```python
from build123d import *

# Parameters (mm, degrees)
W_TOP_DEPTH                  = 3.175
SKETCH3_W                    = 16.4
SKETCH3_H                    = 12
SKETCH3_W_2                  = 35.6
SKETCH3_H_2                  = 4.6
A_HOLDERS_DEPTH              = 5.5
A_CLAMP_DEPTH                = 2
SKETCH12_R                   = 1.35
SKETCH12_W                   = 25
SKETCH12_H                   = 45.3
A_HOLES_DEPTH                = 3.175
A_HOLES_START                = 1
A_HOLES_GUIDE_DEPTH          = 1.5
SKETCH15_R                   = 3.175
TENDON_HOLES_DEPTH           = 3.175
SKETCH16_R                   = 4.675
SKETCH16_R_2                 = 3.175
TUBE_SUPPORT_DEPTH           = 5
SKETCH19_R                   = 3.175
THICKNESS_COMPENSATION_DEPTH = 2.2
SKETCH18_R                   = 5
GEAR_PLACEMENTS_DEPTH        = 1.25
SKETCH20_R                   = 2.155
SCREW_HOLES_DEPTH            = 5.375
SKETCH21_R                   = 3.275
STANDOFF_HOLE_DEPTH          = 2.7


with BuildPart() as part:
    # Sketch1 → w_top (new body)
    with BuildSketch(Plane(origin=(0, 0, 0), x_dir=(1, 0, 0), z_dir=(0, 1, 0))):
        with BuildLine():
            Line((-48, -35), (-48, 30))
            ThreePointArc((-48, 30), (-42.142135624, 44.142135624), (-28, 50))
            Line((-28, 50), (28, 50))
            ThreePointArc((28, 50), (42.142135624, 44.142135624), (48, 30))
            Line((48, 30), (48, -35))
            ThreePointArc((48, -35), (42.142135624, -49.142135624), (28, -55))
            Line((28, -55), (-28, -55))
            ThreePointArc((-28, -55), (-42.142135624, -49.142135624), (-48, -35))
        make_face()
    extrude(amount=W_TOP_DEPTH)

    # Sketch3 → a_holders (add)
    with BuildSketch(Plane(origin=(0, 3.175, 0), x_dir=(1, 0, 0), z_dir=(0, 1, 0))):
        Polygon((0.5, -24.5), (0.5, -34), (41.1, -34), (41.1, -24.5), (33, -24.5), (33, -8.5), (8.6, -8.5), (8.6, -24.5), align=None)
        with Locations((20.8, -18.5)):
            Rectangle(SKETCH3_W, SKETCH3_H, mode=Mode.SUBTRACT)
        with Locations((20.8, -29.25)):
            Rectangle(SKETCH3_W_2, SKETCH3_H_2, mode=Mode.SUBTRACT)
        Polygon((8.6, 26.5), (-8.6, 26.5), (-8.6, 10.5), (-33, 10.5), (-33, 26.5), (-41.1, 26.5), (-41.1, 36), (41.1, 36), (41.1, 26.5), (33, 26.5), (33, 10.5), (8.6, 10.5), align=None)
        with Locations((20.8, 20.5)):
            Rectangle(SKETCH3_W, SKETCH3_H, mode=Mode.SUBTRACT)
        with Locations((-20.8, 20.5)):
            Rectangle(SKETCH3_W, SKETCH3_H, mode=Mode.SUBTRACT)
        with Locations((-20.8, 31.25)):
            Rectangle(SKETCH3_W_2, SKETCH3_H_2, mode=Mode.SUBTRACT)
        with Locations((20.8, 31.25)):
            Rectangle(SKETCH3_W_2, SKETCH3_H_2, mode=Mode.SUBTRACT)
    extrude(amount=A_HOLDERS_DEPTH)

    # Sketch14 → a_clamp (add)
    with BuildSketch(Plane(origin=(0, 8.675, 0), x_dir=(1, 0, 0), z_dir=(0, 1, 0))):
        Polygon((-35.6, 33.55), (-35.6, 36), (-41.1, 36), (-41.1, 26.5), (-35.6, 26.5), (-35.6, 28.95), (-38.6, 28.95), (-38.6, 33.55), align=None)
        Polygon((6, -24.5), (0.5, -24.5), (0.5, -34), (6, -34), (6, -31.55), (3, -31.55), (3, -26.95), (6, -26.95), align=None)
        Polygon((-3, 33.55), (-6, 33.55), (-6, 36), (6, 36), (6, 33.55), (3, 33.55), (3, 28.95), (6, 28.95), (6, 26.5), (-6, 26.5), (-6, 28.95), (-3, 28.95), align=None)
        Polygon((38.6, 33.55), (35.6, 33.55), (35.6, 36), (41.1, 36), (41.1, 26.5), (35.6, 26.5), (35.6, 28.95), (38.6, 28.95), align=None)
        Polygon((35.6, -26.95), (35.6, -24.5), (41.1, -24.5), (41.1, -34), (35.6, -34), (35.6, -31.55), (38.6, -31.55), (38.6, -26.95), align=None)
    extrude(amount=A_CLAMP_DEPTH)

    # Sketch12 → a_holes (cut)
    with BuildSketch(Plane(origin=(0, 3.175, 0), x_dir=(1, 0, 0), z_dir=(0, 1, 0))):
        with Locations((-28.8, -47.8)):
            Circle(SKETCH12_R)
        with Locations((-11.8, -47.8)):
            Circle(SKETCH12_R)
        with Locations((-35.3, -24.5)):
            Circle(SKETCH12_R)
        with Locations((-5.3, -24.5)):
            Circle(SKETCH12_R)
        with Locations((-20.3, -22.45)):
            Rectangle(SKETCH12_W, SKETCH12_H)
    extrude(amount=-A_HOLES_DEPTH, mode=Mode.SUBTRACT)

    # Sketch13 → a_holes guide (cut)
    with BuildSketch(Plane.XZ.offset(A_HOLES_START)):
        with BuildLine():
            Line((-31.6, 47.8), (-31.6, 45.1))
            Line((-31.6, 45.1), (-26, 45.1))
            Line((-26, 45.1), (-26, 47.8))
            ThreePointArc((-26, 47.8), (-28.8, 50.6), (-31.6, 47.8))
        make_face()
        with BuildLine():
            Line((-35.3, 27.3), (-32.8, 27.3))
            Line((-32.8, 27.3), (-32.8, 21.7))
            Line((-32.8, 21.7), (-35.3, 21.7))
            ThreePointArc((-35.3, 21.7), (-38.1, 24.5), (-35.3, 27.3))
        make_face()
        with BuildLine():
            Line((-7.8, 21.7), (-5.3, 21.7))
            ThreePointArc((-5.3, 21.7), (-2.5, 24.5), (-5.3, 27.3))
            Line((-5.3, 27.3), (-7.8, 27.3))
            Line((-7.8, 27.3), (-7.8, 21.7))
        make_face()
        with BuildLine():
            Line((-14.6, 45.1), (-14.6, 47.8))
            ThreePointArc((-14.6, 47.8), (-11.8, 50.6), (-9, 47.8))
            Line((-9, 47.8), (-9, 45.1))
            Line((-9, 45.1), (-14.6, 45.1))
        make_face()
    extrude(amount=-A_HOLES_GUIDE_DEPTH, mode=Mode.SUBTRACT)

    # Sketch15 → tendon holes (cut)
    with BuildSketch(Plane(origin=(0, 3.175, 0), x_dir=(1, 0, 0), z_dir=(0, 1, 0))):
        with Locations((-10.3, 42.17)):
            Circle(SKETCH15_R)
        with Locations((31.3, 42.17)):
            Circle(SKETCH15_R)
        with Locations((10.3, -40.17)):
            Circle(SKETCH15_R)
    extrude(amount=-TENDON_HOLES_DEPTH, mode=Mode.SUBTRACT)

    # Sketch16 → tube_support (add)
    with BuildSketch(Plane(origin=(0, 3.175, 0), x_dir=(1, 0, 0), z_dir=(0, 1, 0))):
        with Locations((-10.3, 42.17)):
            Circle(SKETCH16_R)
        with Locations((-10.3, 42.17)):
            Circle(SKETCH16_R_2, mode=Mode.SUBTRACT)
        with Locations((31.3, 42.17)):
            Circle(SKETCH16_R)
        with Locations((31.3, 42.17)):
            Circle(SKETCH16_R_2, mode=Mode.SUBTRACT)
        with Locations((10.3, -40.17)):
            Circle(SKETCH16_R)
        with Locations((10.3, -40.17)):
            Circle(SKETCH16_R_2, mode=Mode.SUBTRACT)
    extrude(amount=TUBE_SUPPORT_DEPTH)

    # Sketch19 → thickness compensation (add)
    with BuildSketch(Plane.XZ):
        with BuildLine():
            Line((-48, -30), (-48, 35))
            ThreePointArc((-48, 35), (-42.142135624, 49.142135624), (-28, 55))
            Line((-28, 55), (28, 55))
            ThreePointArc((28, 55), (42.142135624, 49.142135624), (48, 35))
            Line((48, 35), (48, -30))
            ThreePointArc((48, -30), (42.142135624, -44.142135624), (28, -50))
            Line((28, -50), (-28, -50))
            ThreePointArc((-28, -50), (-42.142135624, -44.142135624), (-48, -30))
        make_face()
        with Locations((10.3, 40.17)):
            Circle(SKETCH19_R, mode=Mode.SUBTRACT)
        with Locations((-10.3, -42.17)):
            Circle(SKETCH19_R, mode=Mode.SUBTRACT)
        with Locations((31.3, -42.17)):
            Circle(SKETCH19_R, mode=Mode.SUBTRACT)
        with BuildLine():
            Line((-32.8, -0.2), (-7.8, -0.2))
            Line((-7.8, -0.2), (-7.8, 21.7))
            Line((-7.8, 21.7), (-5.3, 21.7))
            ThreePointArc((-5.3, 21.7), (-2.5, 24.5), (-5.3, 27.3))
            Line((-5.3, 27.3), (-7.8, 27.3))
            Line((-7.8, 27.3), (-7.8, 45.1))
            Line((-7.8, 45.1), (-9, 45.1))
            Line((-9, 45.1), (-9, 47.8))
            ThreePointArc((-9, 47.8), (-11.8, 50.6), (-14.6, 47.8))
            Line((-14.6, 47.8), (-14.6, 45.1))
            Line((-14.6, 45.1), (-26, 45.1))
            Line((-26, 45.1), (-26, 47.8))
            ThreePointArc((-26, 47.8), (-28.8, 50.6), (-31.6, 47.8))
            Line((-31.6, 47.8), (-31.6, 45.1))
            Line((-31.6, 45.1), (-32.8, 45.1))
            Line((-32.8, 45.1), (-32.8, 27.3))
            Line((-32.8, 27.3), (-35.3, 27.3))
            ThreePointArc((-35.3, 27.3), (-38.1, 24.5), (-35.3, 21.7))
            Line((-35.3, 21.7), (-32.8, 21.7))
            Line((-32.8, 21.7), (-32.8, -0.2))
        make_face(mode=Mode.SUBTRACT)
    extrude(amount=THICKNESS_COMPENSATION_DEPTH)

    # Sketch18 → gear placements (cut)
    with BuildSketch(Plane.XZ.offset(2.2)):
        with Locations((-3.329437252, -4.970562748)):
            Circle(SKETCH18_R)
        with Locations((10.3, 14.783890932)):
            Circle(SKETCH18_R)
        with Locations((32.995036048, 22.59)):
            Circle(SKETCH18_R)
        with Locations((10.5, -24.585522991)):
            Circle(SKETCH18_R)
    extrude(amount=-GEAR_PLACEMENTS_DEPTH, mode=Mode.SUBTRACT)

    # Sketch20 → screw holes (cut)
    with BuildSketch(Plane.XZ.offset(2.2)):
        with Locations((-42.142135624, -3.5)):
            Circle(SKETCH20_R)
        with Locations((0, -44.142135624)):
            Circle(SKETCH20_R)
        with Locations((42.142135624, -3.5)):
            Circle(SKETCH20_R)
        with Locations((26.142135624, 49.142135624)):
            Circle(SKETCH20_R)
    extrude(amount=-SCREW_HOLES_DEPTH, mode=Mode.SUBTRACT)

    # Sketch21 → standoff hole (cut)
    with BuildSketch(Plane(origin=(0, 3.175, 0), x_dir=(1, 0, 0), z_dir=(0, 1, 0))):
        with Locations((-42.142135624, 3.5)):
            Circle(SKETCH21_R)
        with Locations((42.142135624, 3.5)):
            Circle(SKETCH21_R)
        with Locations((0, 44.142135624)):
            Circle(SKETCH21_R)
        with Locations((26.142135624, -49.142135624)):
            Circle(SKETCH21_R)
    extrude(amount=-STANDOFF_HOLE_DEPTH, mode=Mode.SUBTRACT)


solid = part.part
```
Here's how the part is built. I have some questions about the finished solid (model axes, mm). A direction names the side the tool comes from. Coordinates: 2 decimals unless noted, no trailing zeros. Order: outer loops, then holes, each group sorted by start corner. A loop starts at its lowest first (then second) coordinate and runs counter-clockwise, first axis right, second up.
Item 1: I'm going to push flat-ended pins straight in: pin 1 Ø5 at (y, z) = (6, -13) entering from +X; pin 2 Ø8 at (x, z) = (12.5, 23) entering from +Y (3 decimals); pin 3 Ø1.6 at (x, y) = (-22, 5) entering from +Z. Where does each tip first touch, or does it pass through?
Response values:
pin 1: stops at x = 33
pin 2: stops at y = 8.675
pin 3: stops at z = -10.5
Item 2: Which directions (+Z, -Z, +X, -X, +Y, -Y) give clear straight access to the entire face, cutting with the end or side of a thin tool? Please do faces 1 (the face through (39, 10.675, -31)), 2 (the face through (-35, 0.5, 26)), 3 (the face through (-21, 8.675, -14)), 4 (the face through (-38.6, 7, -31)), 5 (the face through (-0.281, -0.881, -42.005)).
Response values:
face 1: +Z, -Z, +X, -X, +Y
face 2: -Y
face 3: +Z, -Z, +Y
face 4: +Y
face 5: +Y, -Y
Item 3: If we section it at D-D, the plane z = -3.5: List the corners of the cut face in (x, y) for me (3 decimals).
Response values:
outline: (-48, -2.2) - (-44.297, -2.2) - (-44.297, 0.475) - (-45.417, 0.475) - (-45.417, 3.175) - (-48, 3.175) - close; (-39.987, -2.2) - (-8.108, -2.2) - (-8.108, -0.95) - (1.449, -0.95) - (1.449, -2.2) - (39.987, -2.2) - (39.987, 0.475) - (38.867, 0.475) - (38.867, 3.175) - (-38.867, 3.175) - (-38.867, 0.475) - (-39.987, 0.475) - close; (44.297, -2.2) - (48, -2.2) - (48, 3.175) - (45.417, 3.175) - (45.417, 0.475) - (44.297, 0.475) - close
Item 4: Thinking about a two-plate mould opening in X: for faces 6 (the face through (37, 7, -26.5)), 7 (the face through (-41.1, 7, -31)), 8 (the face through (-40.087, -0.881, -2.853)), which applies, pulls with the +X half, pulls with the -X half, needs draft (parallel to the pull), parting line crosses it, or undercut?
Response values:
face 6: needs draft
face 7: pulls with the -X half
face 8: undercut
Item 5: If we section it at C-C, the plane y = 5: Give the number of separate pieces and of enclosed holes in the cut face, then the cut area to 3 significant figures.
Response values:
separate pieces: 5
enclosed holes: 9
area: 1,370 mm2
Item 6: If we section it at A-A, the plane x = -19.5: List the corners of the cut face in (y, z) for me (3 decimals), then the cut area to 3 significant figures.
Response values:
outline: (-2.2, -50) - (3.175, -50) - (3.175, -36) - (8.675, -36) - (8.675, -33.55) - (3.175, -33.55) - (3.175, -28.95) - (8.675, -28.95) - (8.675, -26.5) - (3.175, -26.5) - (3.175, -14.5) - (8.675, -14.5) - (8.675, -10.5) - (3.175, -10.5) - (3.175, -0.2) - (-2.2, -0.2) - close; (-2.2, 45.1) - (3.175, 45.1) - (3.175, 55) - (-2.2, 55) - close
area: 370 mm2
Item 7: I need wall thicknesses on probe 1 along Z at (x, y) = (-28.8, 2); probe 2 along Z at (x, y) = (10, 4.5); probe 3 along Z at (x, y) = (10.5, -1.4). Which ranges of each line are inside material? Lowest first, please.
Response values:
probe 1: z = -49.98 to -0.2, 45.1 to 46.45, 49.15 to 54.98
probe 2: z = -36 to -33.55, -28.95 to -10.5, 8.5 to 26.95, 31.55 to 34, 35.5 to 37.01, 43.33 to 44.84
probe 3: z = -50 to -29.59, -19.59 to 9.79, 19.78 to 37, 43.34 to 55
Item 8: If we section it at B-B, the plane x = 17: List the corners of the cut face in (y, z) for me (3 decimals).
Response values:
outline: (-2.2, -50) - (3.175, -50) - (3.175, -36) - (8.675, -36) - (8.675, -33.55) - (3.175, -33.55) - (3.175, -28.95) - (8.675, -28.95) - (8.675, -26.5) - (3.175, -26.5) - (3.175, -14.5) - (8.675, -14.5) - (8.675, -10.5) - (3.175, -10.5) - (3.175, 8.5) - (8.675, 8.5) - (8.675, 12.5) - (3.175, 12.5) - (3.175, 24.5) - (8.675, 24.5) - (8.675, 26.95) - (3.175, 26.95) - (3.175, 31.55) - (8.675, 31.55) - (8.675, 34) - (3.175, 34) - (3.175, 55) - (-2.2, 55) - close
